```python
from build123d import *

# Parameters (mm, degrees)
F0_W     = 40
F0_H     = 15
F1_DEPTH = 10
F2_D     = 5.25
F3_T     = -1
F5_D     = 5
F5_DEPTH = 2
F5_TIP   = 1.5021515476


with BuildPart() as f1:
    # F0 (on Top) → F1 (new body)
    with BuildSketch(Plane.XY):
        with Locations((20, 7.5)):
            Rectangle(F0_W, F0_H)
    extrude(amount=F1_DEPTH)

    # F2 (through all)
    with Locations(Plane(origin=(0, 0, 0), x_dir=(1, 0, 0), z_dir=(0, 0, -1))):
        with Locations((10, -7.5), (30, -7.5)):
            Hole(F2_D / 2)

    # F3
    f3_openings = [f1.faces().sort_by_distance(p)[0] for p in [
        (20, 15, 5),
        (20, 7.5, 10),
    ]]
    offset(amount=F3_T, openings=f3_openings)

    # F5
    with Locations(Plane.XZ):
        with Locations((4, 5)):
            Hole(F5_D / 2, depth=F5_DEPTH)
            with Locations((0, 0, -(F5_DEPTH + F5_TIP / 2))):  # 118° drill point
                Cone(0, F5_D / 2, F5_TIP, mode=Mode.SUBTRACT)


solid = f1.part
```
Geometry: final body of the model. Coordinates: model frame, mm. A direction names the side the tool comes from. Round coordinates to 2 decimals unless told otherwise and drop trailing zeros. Write each loop counter-clockwise with the first axis right and the second up, starting at its lowest first coordinate (ties: lowest second). Pieces come first, ordered by that corner, then holes. Notation, with made-up numbers: (-21, -12) -> (-1, -12) arc R11 cw to (-1, -1) -> close; hole circle Ø10 at (8, 59). An arc over 180 degrees is marked (long way). Return JSON: item names as keys, results as strings.
Q1. First-contact query: pin 1 Ø4.5 at (x, z) = (18.5, 4.5) entering from +Y. Flat tip, straight axial feed; report the tip coordinate or a pass-through.
From the geometry:
{"pin 1": "y = 1"}
Q2. Set-up query: faces 5 (the cylindrical face through (32.67, 5.05, 5.56)), 6 (the flat face through (39, 8, 5)), 7 (the cylindrical face through (31.935, 5.726, 5.07)). Return all of +Z, -Z, +X, -X, +Y, -Y with unobstructed straight access to the full face (end or side cutting, diameter ignored); none if empty.
From the geometry:
{"face 5": "+Z", "face 6": "+Z, +Y", "face 7": "+Z, -Z"}
Q3. Ray query, line 1 (Y direction, x = 30, z = 6.5) (3 decimals); line 2 (Z direction, x = 4, y = 0.7); line 3 (Y direction, x = 29, z = 4.5). Return the intervals inside material, ascending.
From the geometry:
{"line 1": "0 to 1, 3.875 to 4.875, 10.125 to 11.125", "line 2": "0 to 2.5, 7.5 to 10", "line 3": "0 to 1, 4.02 to 5.07, 9.93 to 10.98"}
Q4. Section A-A on z = 8.5. Return the cut outline in (x, y) (3 decimals).
From the geometry:
{"outline": "(0, 0) -> (40, 0) -> (40, 15) -> (39, 15) -> (39, 1) -> (1, 1) -> (1, 15) -> (0, 15) -> close; circle Ø7.25 at (10, 7.5); circle Ø7.25 at (30, 7.5); hole circle Ø5.25 at (10, 7.5); hole circle Ø5.25 at (30, 7.5)"}
Q5. Mould query, pull axis Y, two halves, no side actions, for faces 1 (the cylindrical face through (10.472, 3.906, 5.563)), 2 (the cylindrical face through (11.935, 5.726, 5.07)), 3 (the flat face through (0, 7, 5)), 4 (the flat face through (19.9, 15, 0.5)). Classes: +Y half, -Y half, draft (parallel to the pull), parting line (faces both ways), or undercut.
From the geometry:
{"face 1": "undercut", "face 2": "undercut", "face 3": "draft", "face 4": "+Y half"}
Q6. Section C-C on x = 30. Return the cut outline in (y, z) (3 decimals), and give its area (4 significant figures).
From the geometry:
{"outline": "(0, 0) -> (4.875, 0) -> (4.875, 10) -> (3.875, 10) -> (3.875, 1) -> (1, 1) -> (1, 10) -> (0, 10) -> close; (10.125, 0) -> (15, 0) -> (15, 1) -> (11.125, 1) -> (11.125, 10) -> (10.125, 10) -> close", "area": "36.75 mm2"}
Q7. Section D-D on y = 6.75. Return the cut outline in (x, z).
From the geometry:
{"outline": "(0, 0) -> (7.48, 0) -> (7.48, 10) -> (6.45, 10) -> (6.45, 1) -> (1, 1) -> (1, 10) -> (0, 10) -> close; (12.52, 0) -> (27.48, 0) -> (27.48, 10) -> (26.45, 10) -> (26.45, 1) -> (13.55, 1) -> (13.55, 10) -> (12.52, 10) -> close; (32.52, 0) -> (40, 0) -> (40, 10) -> (39, 10) -> (39, 1) -> (33.55, 1) -> (33.55, 10) -> (32.52, 10) -> close"}
Q8. Section B-B on z = 6.5. Return the cut outline in (x, y) (3 decimals).
From the geometry:
{"outline": "(0, 0) -> (2, 0) -> (2, 1) -> (1, 1) -> (1, 15) -> (0, 15) -> close; (6, 0) -> (40, 0) -> (40, 15) -> (39, 15) -> (39, 1) -> (6, 1) -> close; circle Ø7.25 at (10, 7.5); circle Ø7.25 at (30, 7.5); hole circle Ø5.25 at (10, 7.5); hole circle Ø5.25 at (30, 7.5)"}
